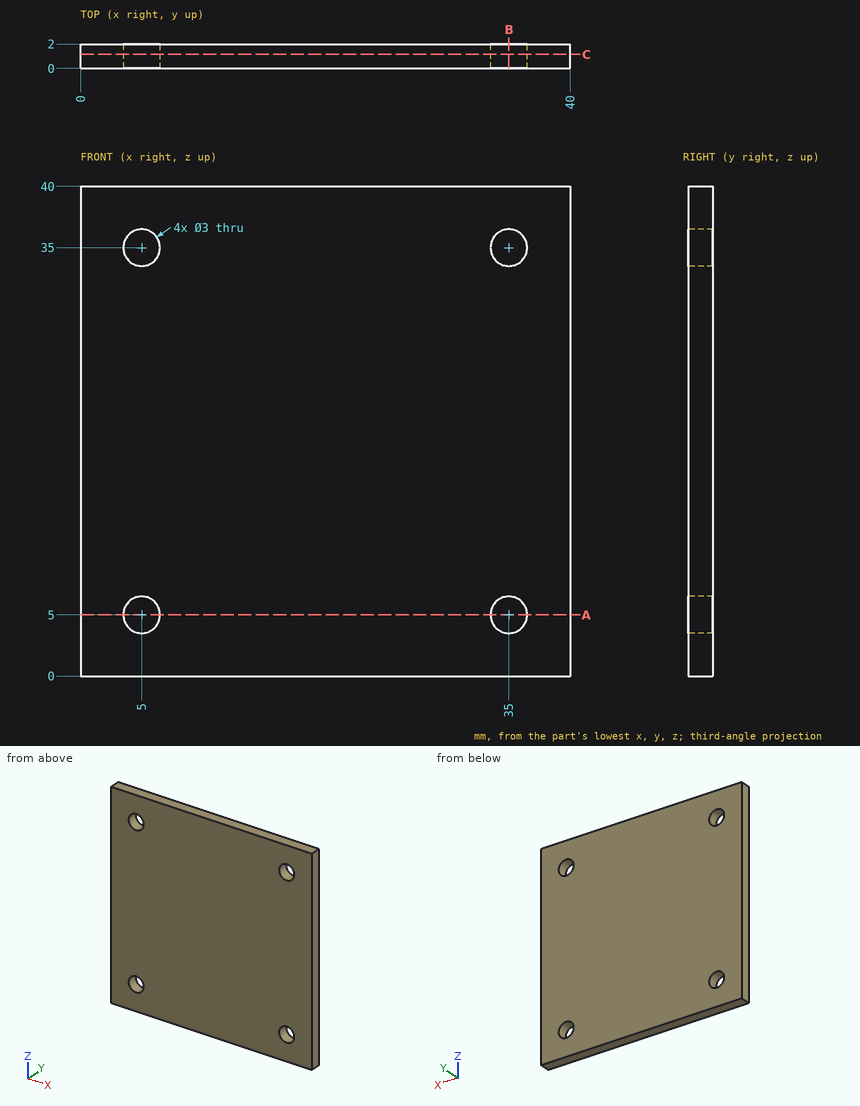
Here's the drawing with two shaded views (mm, measured from the low corner). I have some questions. Give positions to 0.01 mm unless a question says otherwise; leave off trailing zeros. Write each loop counter-clockwise with the first axis right and the second up, starting at its lowest first coordinate (ties: lowest second). Pieces come first, ordered by that corner, then holes. Notation, with made-up numbers: (-36.75, 2) -> (-32.75, 2) arc R7 ccw to (-32.75, 10) -> close; hole circle Ø9 at (57.5, 77.25). An arc over 180 degrees is marked (long way). Answer as a JSON object with one key per item and string values. Group by question number.
Item 1: Suppose I cut it at A-A (z = 5). Please give me the cut outline in (x, y), plus the area to 3 significant figures.
Item 2: I'm going to push a flat-ended pin straight in: P1, Ø2.5, axis at x = 35, z = 35, coming from the -Y side. Where does the tip first touch, or does it pass through?
Item 3: Suppose I cut it at C-C (y = 1.15). Please give me the cut outline in (x, z), plus the area to 3 significant figures.
Item 4: Please list where these lines run through material, in increasing order: line 1 (Z direction, x = 5, y = 0.8); line 2 (Z direction, x = 36, y = 0.85). Write a range as [from, to].
Item 5: Suppose I cut it at B-B (x = 35). Please give me the cut outline in (y, z), plus the area to 3 significant figures.
Findings:
{
 "1": {"outline": "(0, 0) -> (3.5, 0) -> (3.5, 2) -> (0, 2) -> close; (6.5, 0) -> (33.5, 0) -> (33.5, 2) -> (6.5, 2) -> close; (36.5, 0) -> (40, 0) -> (40, 2) -> (36.5, 2) -> close", "area": "68.0 mm²"},
 "2": {"P1": "passes through"},
 "3": {"outline": "(0, 0) -> (40, 0) -> (40, 40) -> (0, 40) -> close; hole circle Ø3 at (5, 5); hole circle Ø3 at (5, 35); hole circle Ø3 at (35, 5); hole circle Ø3 at (35, 35)", "area": "1,570 mm²"},
 "4": {"line 1": "z = [0, 3.5], [6.5, 33.5], [36.5, 40]", "line 2": "z = [0, 3.88], [6.12, 33.88], [36.12, 40]"},
 "5": {"outline": "(0, 0) -> (2, 0) -> (2, 3.5) -> (0, 3.5) -> close; (0, 6.5) -> (2, 6.5) -> (2, 33.5) -> (0, 33.5) -> close; (0, 36.5) -> (2, 36.5) -> (2, 40) -> (0, 40) -> close", "area": "68.0 mm²"}
}
